```python
from build123d import *

# Parameters (mm, degrees)
SKETCH1_R           = 2.5
SKETCH1_R_2         = 1.75
SKETCH1_W           = 46.5
SKETCH1_H           = 6
SKETCH1_R_3         = 1.5
BOSS_EXTRUDE1_DEPTH = 29
SKETCH1_3_W         = 46.5
SKETCH1_3_H         = 6
SKETCH1_3_R         = 1.5
CUT_EXTRUDE1_DEPTH  = 27.5


with BuildPart() as part:
    # Sketch1 → Boss-Extrude1 (new body)
    with BuildSketch(Plane.XY):
        with BuildLine():
            Line((27, 29), (-27, 29))
            ThreePointArc((-27, 29), (-28.414213562, 28.414213562), (-29, 27))
            Line((-29, 27), (-29, -23))
            Line((-29, -23), (17.5, -23))
            Line((17.5, -23), (17.5, -29))
            Line((17.5, -29), (27, -29))
            ThreePointArc((27, -29), (28.414213562, -28.414213562), (29, -27))
            Line((29, -27), (29, 27))
            ThreePointArc((29, 27), (28.414213562, 28.414213562), (27, 29))
        make_face()
        with Locations((23, -14)):
            Circle(SKETCH1_R, mode=Mode.SUBTRACT)
        with Locations((-23, -14)):
            Circle(SKETCH1_R, mode=Mode.SUBTRACT)
        with Locations((25, 25)):
            Circle(SKETCH1_R_2, mode=Mode.SUBTRACT)
        with Locations((-12.5, 23)):
            Circle(SKETCH1_R, mode=Mode.SUBTRACT)
        with Locations((-25, 25)):
            Circle(SKETCH1_R_2, mode=Mode.SUBTRACT)
        with Locations((-5.75, -26)):
            Rectangle(SKETCH1_W, SKETCH1_H)
        with Locations((11, -26)):
            Circle(SKETCH1_R_3, mode=Mode.SUBTRACT)
        with Locations((-23, -26)):
            Circle(SKETCH1_R_3, mode=Mode.SUBTRACT)
    extrude(amount=BOSS_EXTRUDE1_DEPTH)

    # Sketch1_3 → Cut-Extrude1 (cut)
    with BuildSketch(Plane.XY):
        with Locations((-5.75, -26)):
            Rectangle(SKETCH1_3_W, SKETCH1_3_H)
        with Locations((11, -26)):
            Circle(SKETCH1_3_R, mode=Mode.SUBTRACT)
        with Locations((-23, -26)):
            Circle(SKETCH1_3_R, mode=Mode.SUBTRACT)
    extrude(amount=CUT_EXTRUDE1_DEPTH, mode=Mode.SUBTRACT)


solid = part.part
```
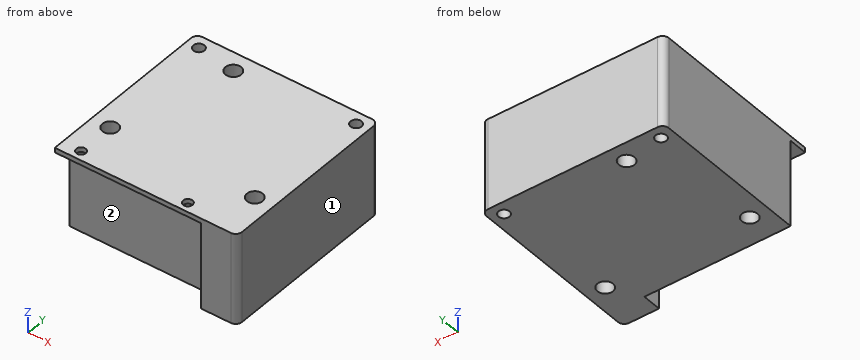
The listing builds one solid part. Answer for the finished solid, in the listing's coordinates (mm). Face numbers are marked on the shaded views. A direction names the side the tool comes from. Coordinates: 2 decimals unless noted, no trailing zeros. Order: outer loops, then holes, each group sorted by start corner. A loop starts at its lowest first (then second) coordinate and runs counter-clockwise, first axis right, second up. Notation, with made-up numbers: M -7.5,2.25 L 44.5,2.25 A26 ccw 44.5,31.25 Z; hole C -7,0 d11. An arc over 180 degrees is marked long. Answer as a JSON object with one key per item and string values. Group by question number.
1. Flat-ended cylindrical pins translate along their axes: P1, Ø14, axis at x = -14.5, z = 19.5, coming from the -Y side; P2, Ø1.8, axis at x = -10.5, y = -27, coming from the -Z side; P3, Ø3, axis at y = -26.5, z = 17.5, coming from the -X side. Find the tip coordinate at first contact, or state that the pin passes through.
2. Section D-D on x = 11 is taken. Write down the section's boundary in (y, z).
3. Section C-C on z = 3.75 is taken. Write down the section's boundary in (x, y), then the cut area to 3 significant figures.
4. Section A-A on y = -26 is taken. Write down the section's boundary in (x, z).
5. A tool of negligible diameter and unlimited length cuts with its end or side. For the marked faces 1 and 2, from which of +Z, -Z, +X, -X, +Y, -Y can it reach the whole face along a straight path? Write none if from no direction.
6. Section B-B on x = -12.5 is taken. Write down the section's boundary in (y, z), then the cut area to 3 significant figures.
7. Straight lines are drawn through the part: line 1 (Y direction, x = -23, z = 28.15); line 2 (Y direction, x = 11, z = 28.1); line 3 (X direction, y = -12, z = 3.25). For each, find the intervals that lie inside material, in ascending order.
Values follow:
{
 "1": {"P1": "y = -23", "P2": "z = 27.5", "P3": "x = 17.5"},
 "2": {"outline": "M -29,27.5 L -27.5,27.5 L -27.5,29 L -29,29 Z; M -24.5,27.5 L -23,27.5 L -23,0 L 29,0 L 29,29 L -24.5,29 Z"},
 "3": {"outline": "M -29,-23 L 17.5,-23 L 17.5,-29 L 27,-29 A2 ccw 29,-27 L 29,27 A2 ccw 27,29 L -27,29 A2 ccw -29,27 Z; hole C -25,25 d3.5; hole C -23,-14 d5; hole C -12.5,23 d5; hole C 23,-14 d5; hole C 25,25 d3.5", "area": "3,000 mm2"},
 "4": {"outline": "M -29,27.5 L -24.5,27.5 L -24.5,29 L -29,29 Z; M -21.5,27.5 L 9.5,27.5 L 9.5,29 L -21.5,29 Z; M 12.5,27.5 L 17.5,27.5 L 17.5,0 L 29,0 L 29,29 L 12.5,29 Z"},
 "5": {"face 1": "+Z, -Z, +X, +Y, -Y", "face 2": "-Z, -X, -Y"},
 "6": {"outline": "M -29,27.5 L -23,27.5 L -23,0 L 20.5,0 L 20.5,29 L -29,29 Z; M 25.5,0 L 29,0 L 29,29 L 25.5,29 Z", "area": "1,370 mm2"},
 "7": {"line 1": "-29 to -27.5, -24.5 to -16.5, -11.5 to 29", "line 2": "-29 to -27.5, -24.5 to 29", "line 3": "-29 to -24.5, -21.5 to 21.5, 24.5 to 29"}
}
